The drawing under review shows one solid part. Ordinate dimensions are in mm from its lowest x, y, z. A direction names the side the tool comes from. Coordinates: 2 decimals unless noted, no trailing zeros. Write each loop counter-clockwise with the first axis right and the second up, starting at its lowest first coordinate (ties: lowest second). Pieces come first, ordered by that corner, then holes.
1) We need section C-C on y = 2.75. Give the number of separate pieces and of enclosed holes in the cut face, then the cut area to 3 significant figures.
2) Mouldability with a two-part tool opening along X and no side actions: class the marked faces 3, 4, 5 and 6 as pulls with the +X half, pulls with the -X half, needs draft (parallel to the pull), parting line crosses it, or undercut.
3) We need section D-D on x = 14. Write out the cut boundary in (y, z) (1 decimal), then the cut area to 3 significant figures.
4) Insertion check: P1, Ø3, axis at y = 6, z = 4, coming from the +X side (1 decimal); P2, Ø3, axis at x = 6, z = 6.5, coming from the +Y side (1 decimal). Each pin has a flat end and moves straight along its axis. Give the tip position at first contact, or say it passes through.
5) To check wall thickness, follow line 1 along Y through (x, z) = (12.7, 6) (1 decimal); line 2 along Y through (x, z) = (23.5, 4) (1 decimal); line 3 along X through (y, z) = (7.75, 0.5) (1 decimal). State the ranges of each line that lie inside material, in increasing order.
6) For the marked faces 1 and 2, list the 3-axis set-ups (+Z, -Z, +X, -X, +Y, -Y) from which the entire face can be reached by the end or side of a thin tool; tool diameter is ignored.
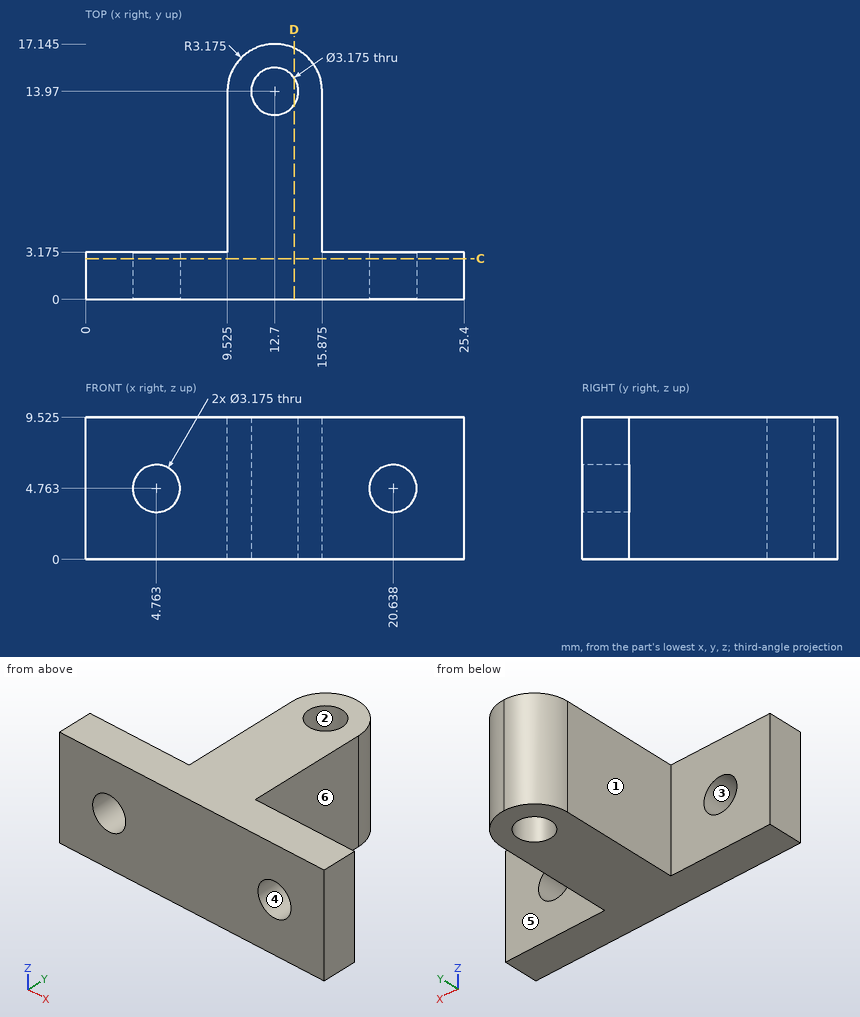
Result:
1. separate pieces: 1
1. enclosed holes: 2
1. area: 226 mm2
2. face 3: undercut
2. face 4: undercut
2. face 5: needs draft
2. face 6: pulls with the +X half
3. outline: (0, 0) - (13.1, 0) - (13.1, 9.5) - (0, 9.5) - close; (14.9, 0) - (16.9, 0) - (16.9, 9.5) - (14.9, 9.5) - close
3. area: 143 mm2
4. P1: stops at x = 15.9
4. P2: stops at y = 3.2
5. line 1: y = 0 to 12.4, 15.6 to 17.1
5. line 2: y = 0 to 3.2
5. line 3: x = 9.5 to 15.9
6. face 1: +Z, -Z, -X, +Y
6. face 2: +Z, -Z
